```python
from build123d import *

# Parameters (mm, degrees)
SKETCH1_R               = 7
SKETCH1_R_2             = 4
BOSS_EXTRUDE1_DEPTH     = 10
CUT_EXTRUDE1_DEPTH      = 15.071247279
CUT_EXTRUDE1_DEPTH_BACK = 15.071247279
SKETCH2_R               = 2
CHAMFER1_SIZE           = 1


with BuildPart() as part:
    # Sketch1 → Boss-Extrude1 (new, symmetric)
    with BuildSketch(Plane(origin=(0, 0, 0), x_dir=(0, 0, -1), z_dir=(1, 0, 0))):
        Circle(SKETCH1_R)
        Circle(SKETCH1_R_2, mode=Mode.SUBTRACT)
    extrude(amount=BOSS_EXTRUDE1_DEPTH, both=True)

    # Sketch2 → Cut-Extrude1 (cut, two sides: drawn at the far end of the back side and taken through both)
    with BuildSketch(Plane(origin=(0, 0, 0), x_dir=(1, 0, 0), z_dir=(0, 1, 0)).offset(-CUT_EXTRUDE1_DEPTH_BACK)):
        with Locations(Location((-6, 0, 0), (0, 0, 270))):
            Circle(SKETCH2_R)
        with Locations(Location((6, 0, 0), (0, 0, 270))):
            Circle(SKETCH2_R)
    extrude(amount=CUT_EXTRUDE1_DEPTH + CUT_EXTRUDE1_DEPTH_BACK, mode=Mode.SUBTRACT)

    # Chamfer1
    chamfer1_edges = [part.edges().sort_by_distance(p)[0] for p in [
        (-10, 0, 7),
        (10, 0, 7),
    ]]
    chamfer(chamfer1_edges, length=CHAMFER1_SIZE)


solid = part.part
```
Design review of the part built by this model. Coordinates are the model's own, in mm. Give positions to 0.01 mm unless a question says otherwise; leave off trailing zeros. Order: outer loops, then holes, each group sorted by start corner. A loop starts at its lowest first (then second) coordinate and runs counter-clockwise, first axis right, second up. Notation, with made-up numbers: (-37, 32.5) -> (15, 32.5) arc R29 cw to (15, 55.5) -> close; hole circle Ø3 at (42.5, 75.5). An arc over 180 degrees is marked (long way). Write each question's results on one line, items separated by ' | '. Start each with the question number.
Q1. Wall thickness on L1, parallel to X at y = -4.4, z = 0; L2, parallel to Z at x = 6, y = -4.9; L3, parallel to Y at x = 3.75, z = -2.75: over which ranges is each line inside the solid? List them lowest first. Write a range as from..to.
Q2. Add section C-C on x = 6.75. Give the boundary of the cut face in (y, z).
Q3. Add section D-D on y = 5.75. State how many separate pieces and enclosed holes the cut face has, and give its area (3 significant figures).
Q4. Add section A-A on y = 0. Give the boundary of the cut face in (x, z).
Q5. Mouldability with a two-part tool opening along X and no side actions: class faces 1 (the cylindrical face through (-8, 5, 0)), 2 (the flat face through (-10, -3.92, 1.42)), 3 (the flat face through (10, -3.92, 1.42)) as +X half, -X half, draft (parallel to the pull), parting line (faces both ways), or undercut.
Q6. Add section B-B on z = 0. Give the boundary of the cut face in (x, y), and give its area (3 significant figures).
Q7. For pin 1 (2 mm diameter, centred on x = -6.5, y = 4, fed in from +Z); pin 2 (3 mm diameter, centred on x = 6, z = 2, fed in from +Y); pin 3 (2 mm diameter, centred on x = 0, z = -2.5, fed in from -Y), all flat-tipped, find the tip position at first contact; note any pin that passes through.
Found:
1) L1: x = -10..-8, -4..4, 8..10 | L2: z = -5..-2, 2..5 | L3: y = -6.44..-2.9, 2.9..6.44
2) outline: (-6.75, -1.85) arc R7 ccw to (6.75, -1.85) -> (3.54, -1.85) arc R4 cw to (-3.54, -1.85) -> close; (-6.75, 1.85) -> (-3.54, 1.85) arc R4 cw to (3.54, 1.85) -> (6.75, 1.85) arc R7 ccw to start
3) separate pieces: 1 | enclosed holes: 2 | area: 130 mm2
4) outline: (-10, -6) -> (-9, -7) -> (9, -7) -> (10, -6) -> (10, -4) -> (-10, -4) -> close; (-10, 4) -> (10, 4) -> (10, 6) -> (9, 7) -> (-9, 7) -> (-10, 6) -> close
5) face 1: undercut | face 2: -X half | face 3: +X half
6) outline: (-10, -6) -> (-9, -7) -> (-8, -7) -> (-8, -4) -> (-10, -4) -> close; (-10, 4) -> (-8, 4) -> (-8, 7) -> (-9, 7) -> (-10, 6) -> close; (-4, -7) -> (4, -7) -> (4, -4) -> (-4, -4) -> close; (-4, 4) -> (4, 4) -> (4, 7) -> (-4, 7) -> close; (8, -7) -> (9, -7) -> (10, -6) -> (10, -4) -> (8, -4) -> close; (8, 4) -> (10, 4) -> (10, 6) -> (9, 7) -> (8, 7) -> close | area: 70.0 mm2
7) pin 1: stops at z = 6.32 | pin 2: stops at y = 6.85 | pin 3: stops at y = -6.84
